Check sheet for the modelled part. Datum: model origin and axes. Units: mm. Give positions to 0.01 mm unless a question says otherwise; leave off trailing zeros. Write each loop counter-clockwise with the first axis right and the second up, starting at its lowest first coordinate (ties: lowest second). Pieces come first, ordered by that corner, then holes. Notation, with made-up numbers: M -21.75,65 L 14.25,65 A14 ccw 14.25,74 Z; hole C 59,55 d7. An arc over 180 degrees is marked long. Use CSV: the item, a comma, the result in double quotes. Start each with the question number.
1. Scan lines: line 1 (Y direction, x = -0.4, z = 0); line 2 (Z direction, x = 0.6, y = 1); line 3 (Y direction, x = -0.7, z = 2). Record each from-to range of solid material in increasing order.
2. Cross-section at C-C, the plane x = -0.6. State how many separate pieces and enclosed holes the cut face has, and give its area (3 significant figures).
3. Cross-section at B-B, the plane y = -13. Enter the section's corners in (x, z).
4. Cross-section at D-D, the plane y = 15. Enter the section's corners in (x, z).
5. Depth check by flat-ended pin: P1, Ø1, axis at x = -1.5, y = -3, coming from the +Z side. Enter the tip coordinate at first touch or a pass-through.
6. Cross-section at A-A, the plane z = 0. Enter the section's corners in (x, y).
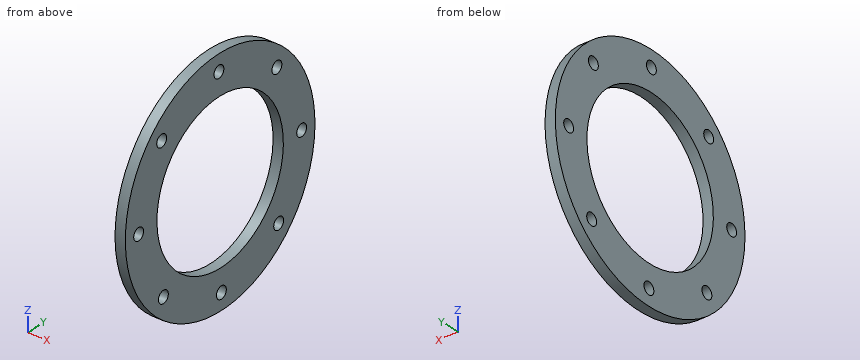
from build123d import *

# Parameters (mm, degrees)
SKETCH3_W          = 4
SKETCH3_H          = 15
SKETCH4_R          = 2.339551022
CUT_EXTRUDE1_DEPTH = 4


with BuildPart() as part:
    # Sketch3 → Revolve1 (revolve)
    with BuildSketch(Plane.XY, mode=Mode.PRIVATE) as revolve1_sk:
        with Locations((0, 37.5)):
            Rectangle(SKETCH3_W, SKETCH3_H)
    revolve(revolve1_sk.sketch.rotate(Axis((0, 0, 0), (1, 0, 0)), 90), axis=Axis((0, 0, 0), (1, 0, 0)))

    # Sketch4 → Cut-Extrude1 (cut)
    with BuildSketch(Plane.ZY.offset(2)):
        with Locations((0.585786438, 38.689785425)):
            Circle(SKETCH4_R)
        with Locations((27.772023199, 26.943596075)):
            Circle(SKETCH4_R)
        with Locations((38.689785425, -0.585786438)):
            Circle(SKETCH4_R)
        with Locations((26.943596075, -27.772023199)):
            Circle(SKETCH4_R)
        with Locations((-0.585786438, -38.689785425)):
            Circle(SKETCH4_R)
        with Locations((-27.772023199, -26.943596075)):
            Circle(SKETCH4_R)
        with Locations((-38.689785425, 0.585786438)):
            Circle(SKETCH4_R)
        with Locations((-26.943596075, 27.772023199)):
            Circle(SKETCH4_R)
    extrude(amount=-CUT_EXTRUDE1_DEPTH, mode=Mode.SUBTRACT)


solid = part.part
Worked answers:
1,line 1,"y = -45 to -40.95, -36.42 to -30, 30 to 36.42, 40.95 to 45"
1,line 2,"z = -44.99 to -40.99, -36.39 to -29.98, 29.98 to 36.97, 40.41 to 44.99"
1,line 3,"y = -44.96 to -29.93, 29.93 to 36.83, 40.55 to 44.96"
2,separate pieces,"1"
2,enclosed holes,"9"
2,area,"3,400 mm^2"
3,outline,"M -2,-43.08 L 2,-43.08 L 2,-27.04 L -2,-27.04 Z; M -2,27.04 L 2,27.04 L 2,43.08 L -2,43.08 Z"
4,outline,"M -2,-42.43 L 2,-42.43 L 2,-25.98 L -2,-25.98 Z; M -2,25.98 L 2,25.98 L 2,42.43 L -2,42.43 Z"
5,P1,"stops at z = 44.93"
6,outline,"M -2,-45 L 2,-45 L 2,-40.95 L -2,-40.95 Z; M -2,-36.42 L 2,-36.42 L 2,-30 L -2,-30 Z; M -2,30 L 2,30 L 2,36.42 L -2,36.42 Z; M -2,40.95 L 2,40.95 L 2,45 L -2,45 Z"
